For this review, use the dimensioned drawing (mm, ordinates from the lowest corner) and the shaded views. Round coordinates to 2 decimals unless told otherwise and drop trailing zeros. Write each loop counter-clockwise with the first axis right and the second up, starting at its lowest first coordinate (ties: lowest second). Pieces come first, ordered by that corner, then holes. Notation, with made-up numbers: M 41,-21.5 L 84,-21.5 A32 ccw 84,6.5 Z; hole C 68.25,-0.5 d1. An arc over 180 degrees is marked long. Answer in a Markdown table with one row per item.
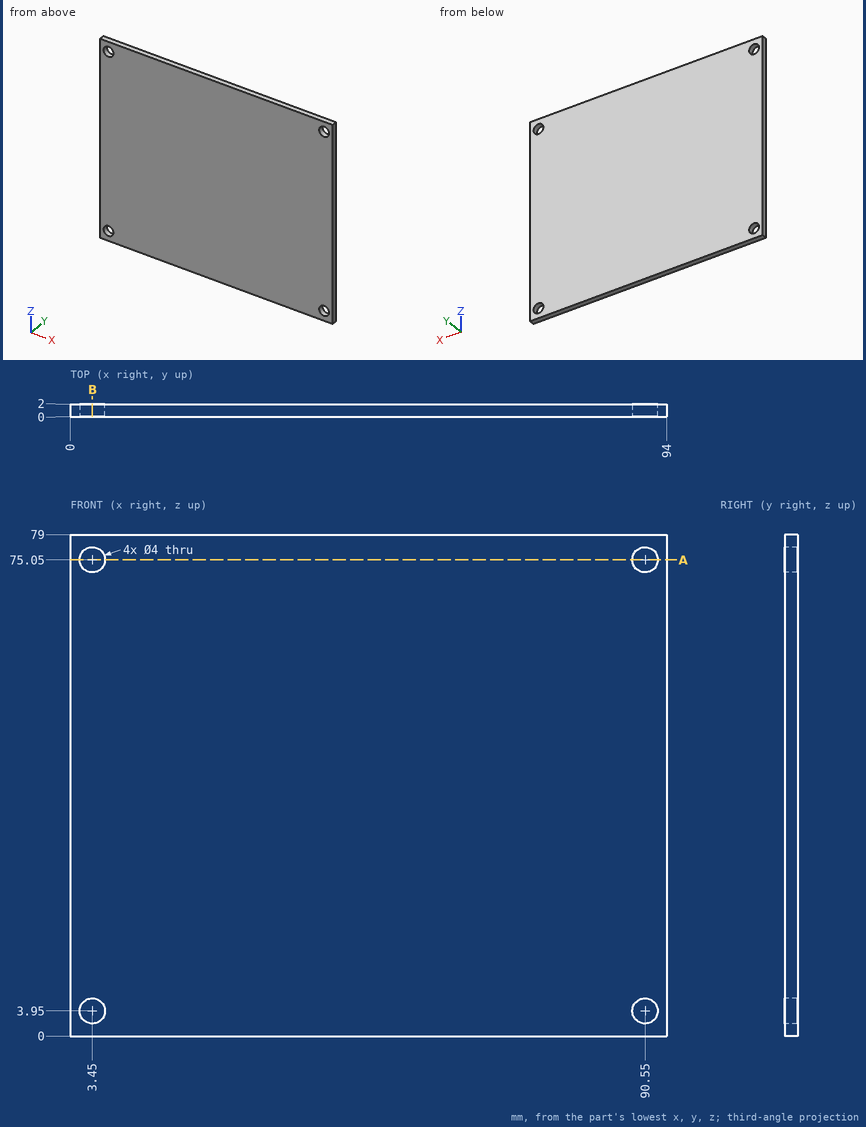
Q1. For probe 1 along Z at (x, y) = (90.55, 1.5); probe 2 along X at (y, z) = (1.4, 75.05); probe 3 along Z at (x, y) = (4.5, 1.85), list the stretches that pass through material, from the lowest coordinate up.
Found:
| item | result |
|---|---|
| probe 1 | 0 to 1.95, 5.95 to 73.05, 77.05 to 79 |
| probe 2 | 0 to 1.45, 5.45 to 88.55, 92.55 to 94 |
| probe 3 | 0 to 2.25, 5.65 to 73.35, 76.75 to 79 |
Q2. Take a section at A-A (z = 75.05). State the section outline as (x, y) points, then the cut area to 3 significant figures.
Found:
| item | result |
|---|---|
| outline | M 0,0 L 1.45,0 L 1.45,2 L 0,2 Z; M 5.45,0 L 88.55,0 L 88.55,2 L 5.45,2 Z; M 92.55,0 L 94,0 L 94,2 L 92.55,2 Z |
| area | 172 mm² |
Q3. Insertion check: P1, Ø3, axis at x = 3.45, z = 3.95, coming from the +Y side. The pin has a flat end and moves straight along its axis. Give the tip position at first contact, or say it passes through.
Found:
| item | result |
|---|---|
| P1 | through |
Q4. Take a section at B-B (x = 3.45). State the section outline as (y, z) points.
Found:
| item | result |
|---|---|
| outline | M 0,0 L 2,0 L 2,1.95 L 0,1.95 Z; M 0,5.95 L 2,5.95 L 2,73.05 L 0,73.05 Z; M 0,77.05 L 2,77.05 L 2,79 L 0,79 Z |
